Could you check a few things on this drawing? It's one solid part, dimensions in mm from its lowest x, y, z. A direction names the side the tool comes from. Give positions to 0.01 mm unless a question says otherwise; leave off trailing zeros. Order: outer loops, then holes, each group sorted by start corner. A loop starts at its lowest first (then second) coordinate and runs counter-clockwise, first axis right, second up. Notation, with made-up numbers: (68, 76.25) -> (79, 76.25) arc R13 cw to (79, 83.25) -> close; hole circle Ø7 at (39, -18.5). An arc over 180 degrees is marked (long way). Answer as a JSON object with one key per item and string values.
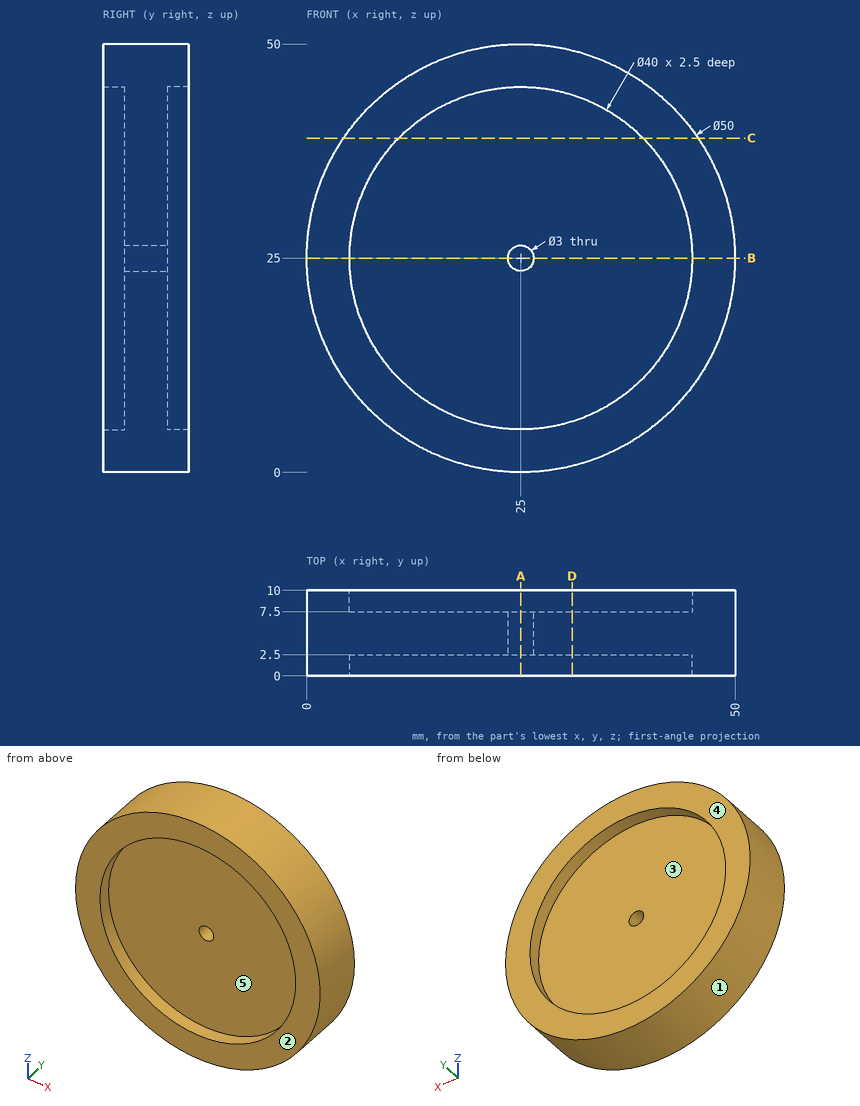
1. If we section it at A-A on x = 25: Please give me the cut outline in (y, z), then the cut area to 3 significant figures.
Worked answers:
{"outline": "(0, 0) -> (10, 0) -> (10, 5) -> (7.5, 5) -> (7.5, 23.5) -> (2.5, 23.5) -> (2.5, 5) -> (0, 5) -> close; (0, 45) -> (2.5, 45) -> (2.5, 26.5) -> (7.5, 26.5) -> (7.5, 45) -> (10, 45) -> (10, 50) -> (0, 50) -> close", "area": "285 mm²"}
2. If we section it at B-B on z = 25: Please give me the cut outline in (x, y), then the cut area to 3 significant figures.
Worked answers:
{"outline": "(0, 0) -> (5, 0) -> (5, 2.5) -> (23.5, 2.5) -> (23.5, 7.5) -> (5, 7.5) -> (5, 10) -> (0, 10) -> close; (26.5, 2.5) -> (45, 2.5) -> (45, 0) -> (50, 0) -> (50, 10) -> (45, 10) -> (45, 7.5) -> (26.5, 7.5) -> close", "area": "285 mm²"}
3. If we section it at D-D on x = 31: Please give me the cut outline in (y, z).
Worked answers:
{"outline": "(0, 0.73) -> (10, 0.73) -> (10, 5.92) -> (7.5, 5.92) -> (7.5, 44.08) -> (10, 44.08) -> (10, 49.27) -> (0, 49.27) -> (0, 44.08) -> (2.5, 44.08) -> (2.5, 5.92) -> (0, 5.92) -> close"}
4. If we section it at C-C on z = 39: Please give me the cut outline in (x, y), then the cut area to 3 significant figures.
Worked answers:
{"outline": "(4.29, 0) -> (10.72, 0) -> (10.72, 2.5) -> (39.28, 2.5) -> (39.28, 0) -> (45.71, 0) -> (45.71, 10) -> (39.28, 10) -> (39.28, 7.5) -> (10.72, 7.5) -> (10.72, 10) -> (4.29, 10) -> close", "area": "271 mm²"}
5. Will these pins go through, and if not, where does the flat tip stop? pin 1 Ø5 at (x, z) = (25, 25) entering from +Y; pin 2 Ø6 at (x, y) = (26.5, 5.5) entering from +Z; pin 3 Ø1 at (x, z) = (39, 15.5) entering from -Y.
Worked answers:
{"pin 1": "y = 7.5", "pin 2": "z = 50", "pin 3": "y = 2.5"}
6. If we mould it in two halves opening along Z, with no side actions, what happens to the marked faces 1, 2 and 3? For each: +Z half, -Z half, draft (parallel to the pull), parting line (faces both ways), or undercut.
Worked answers:
{"face 1": "parting line", "face 2": "draft", "face 3": "undercut"}
7. For the marked faces 4 and 5, which set-ups out of +Z, -Z, +X, -X, +Y, -Y let a thin tool reach every point of the face, with its end or its side?
Worked answers:
{"face 4": "+Z, -Z, +X, -X, +Y", "face 5": "-Y"}
8. Please list where these lines run through material, in increasing order: L1, parallel to Z at x = 25, y = 9.15; L2, parallel to Y at x = 42.5, z = 15.5; L3, parallel to Z at x = 25, y = 4.6.
Worked answers:
{"L1": "0 to 5, 45 to 50", "L2": "2.5 to 7.5", "L3": "0 to 23.5, 26.5 to 50"}
